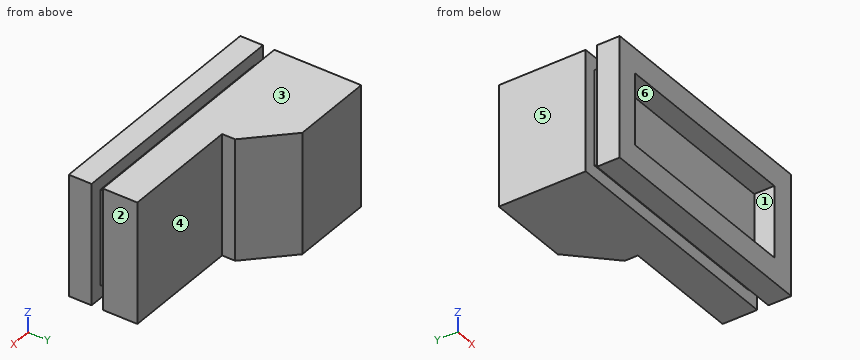
```python
from build123d import *

# Parameters (mm, degrees)
BOSS_EXTRUDE1_DEPTH = 25.4
SKETCH2_W           = 101.6
SKETCH2_H           = 50.8
SKETCH2_W_2         = 90.88
SKETCH2_H_2         = 40.08
CUT_EXTRUDE1_DEPTH  = 4.72
SKETCH3_W           = 82.6
SKETCH3_H           = 30
CUT_EXTRUDE2_DEPTH  = 8.43


with BuildPart() as part:
    # Sketch1 → Boss-Extrude1 (new, symmetric)
    with BuildSketch(Plane.XY):
        Polygon((0, 0), (0, 50.8), (34.9, 50.8), (51.39, 34.31), (51.39, 28.81), (101.6, 28.81), (101.6, 0), align=None)
    extrude(amount=BOSS_EXTRUDE1_DEPTH, both=True)

    # Sketch2 → Cut-Extrude1 (cut)
    with BuildSketch(Plane(origin=(0, 9.57, 0), x_dir=(-1, 0, 0), z_dir=(0, -1, 0))):
        with Locations((-50.8, 0)):
            Rectangle(SKETCH2_W, SKETCH2_H)
        with Locations((-50.8, 0)):
            Rectangle(SKETCH2_W_2, SKETCH2_H_2, mode=Mode.SUBTRACT)
    extrude(amount=-CUT_EXTRUDE1_DEPTH, mode=Mode.SUBTRACT)

    # Sketch3 → Cut-Extrude2 (cut)
    with BuildSketch(Plane.XZ):
        with Locations((50.3, 0)):
            Rectangle(SKETCH3_W, SKETCH3_H)
    extrude(amount=-CUT_EXTRUDE2_DEPTH, mode=Mode.SUBTRACT)


solid = part.part
```
Design review of the part built by this model. Coordinates are the model's own, in mm. Face numbers are marked on the shaded views. A direction names the side the tool comes from. Round coordinates to 2 decimals unless told otherwise and drop trailing zeros. Write each loop counter-clockwise with the first axis right and the second up, starting at its lowest first coordinate (ties: lowest second). Pieces come first, ordered by that corner, then holes.
Item 1: For the marked faces 4, 5 and 6, list the 3-axis set-ups (+Z, -Z, +X, -X, +Y, -Y) from which the entire face can be reached by the end or side of a thin tool; tool diameter is ignored.
Item 2: We need section D-D on z = -2. Write out the cut boundary in (x, y), and give its area (3 significant figures).
Item 3: We need section B-B on x = 23. Write out the cut boundary in (y, z).
Item 4: Clearance check with flat-ended pins moving along their axes: pin 1 Ø9 at (x, z) = (53.5, 3.5) entering from -Y; pin 2 Ø4 at (y, z) = (31.5, 2) entering from +X; pin 3 Ø2.5 at (x, y) = (47, 12) entering from +Z. State where each tip first meets the part, or that it passes through.
Item 5: We need section C-C on y = 3. Write out the cut boundary in (x, z).
Item 6: For probe 1 along X at (y, z) = (7, 4); probe 2 along Y at (x, z) = (97.5, 3.5); probe 3 along Y at (x, z) = (90, -2), list the stretches that pass through material, from the lowest coordinate up.
Item 7: The part is to be moulded in two halves that separate along Z. For the marked faces 1, 2 and 3, say which applies: +Z half, -Z half, draft (parallel to the pull), parting line (faces both ways), or undercut.
Item 8: We need section A-A on z = 21.5. Write out the cut boundary in (x, y).
Returned:
1. face 4: +Z, -Z, +X, +Y
1. face 5: +Z, -Z, -X, +Y, -Y
1. face 6: -Y
2. outline: (0, 0) - (9, 0) - (9, 8.43) - (91.6, 8.43) - (91.6, 0) - (101.6, 0) - (101.6, 9.57) - (96.24, 9.57) - (96.24, 14.29) - (101.6, 14.29) - (101.6, 28.81) - (51.39, 28.81) - (51.39, 34.31) - (34.9, 50.8) - (0, 50.8) - (0, 14.29) - (5.36, 14.29) - (5.36, 9.57) - (0, 9.57) - close
2. area: 3,170 mm2
3. outline: (0, -25.4) - (9.57, -25.4) - (9.57, -20.04) - (14.29, -20.04) - (14.29, -25.4) - (50.8, -25.4) - (50.8, 25.4) - (14.29, 25.4) - (14.29, 20.04) - (9.57, 20.04) - (9.57, 25.4) - (0, 25.4) - (0, 15) - (8.43, 15) - (8.43, -15) - (0, -15) - close
4. pin 1: stops at y = 8.43
4. pin 2: stops at x = 51.39
4. pin 3: stops at z = 20.04
5. outline: (0, -25.4) - (101.6, -25.4) - (101.6, 25.4) - (0, 25.4) - close; hole (9, -15) - (91.6, -15) - (91.6, 15) - (9, 15) - close
6. probe 1: x = 0 to 9, 91.6 to 101.6
6. probe 2: y = 0 to 9.57, 14.29 to 28.81
6. probe 3: y = 8.43 to 28.81
7. face 1: undercut
7. face 2: draft
7. face 3: +Z half
8. outline: (0, 0) - (101.6, 0) - (101.6, 9.57) - (0, 9.57) - close; (0, 14.29) - (101.6, 14.29) - (101.6, 28.81) - (51.39, 28.81) - (51.39, 34.31) - (34.9, 50.8) - (0, 50.8) - close
